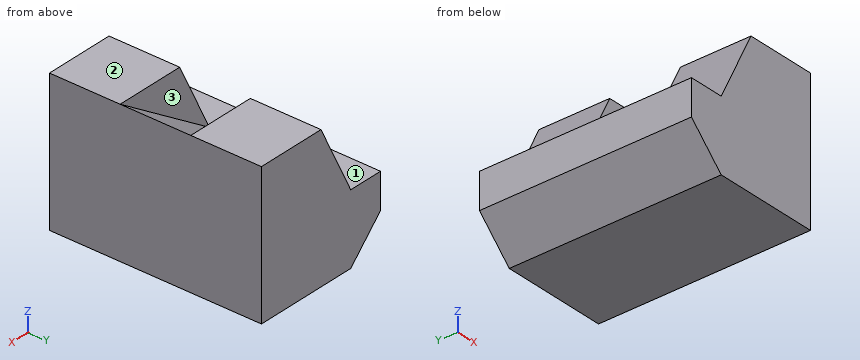
```python
from build123d import *

# Parameters (mm, degrees)
F1_DEPTH = 15
F2_DEPTH = 5


with BuildPart() as f1:
    # F0 (on Front) → F1 (new body, symmetric)
    with BuildSketch(Plane.XZ):
        Polygon((-15, 0), (0, 0), (0, 20), (-15, 10), (-20, 10), (-20, 5), align=None)
        Polygon((-15, 10), (0, 20), (-10, 20), align=None)
    extrude(amount=F1_DEPTH, both=True)

    # F0 (on Front) → F2 (cut, symmetric)
    with BuildSketch(Plane.XZ):
        Polygon((-15, 10), (0, 20), (-10, 20), align=None)
    extrude(amount=F2_DEPTH, both=True, mode=Mode.SUBTRACT)


solid = f1.part
```
Work out the finished part from the listing and answer in its coordinate system (mm). Face numbers are marked on the shaded views. A direction names the side the tool comes from. Round coordinates to 2 decimals unless told otherwise and drop trailing zeros. Write each loop counter-clockwise with the first axis right and the second up, starting at its lowest first coordinate (ties: lowest second). Pieces come first, ordered by that corner, then holes. Notation, with made-up numbers: (35.25, 56.25) - (88.25, 56.25) arc R9 cw to (88.25, 69.25) - close; hole circle Ø4 at (85, -27.75). An arc over 180 degrees is marked (long way). Return JSON: item names as keys, results as strings. Group by question number.
Q1. For the marked faces 1, 2 and 3, determine the directions among +Z, -Z, +X, -X, +Y, -Y from which every point of the face is accessible in a straight line to the end or side of a thin tool.
Q2. Find the intervals of material crossed by L1, parallel to Y at x = -11.5, z = 15.5; L2, parallel to Z at x = -16.75, y = -11; L3, parallel to X at y = -4.5, z = 15.5, in increasing order.
Q3. The part is cut by section D-D on y = -2.75. Write down the section's boundary in (x, z), then the cut area to 4 significant figures.
Q4. The part is cut by section C-C on x = -4.5. Write down the section's boundary in (y, z).
Q5. The part is cut by section B-B on z = 12. Write down the section's boundary in (x, y), then the cut area to 3 significant figures.
Q6. The part is cut by section A-A on y = -8.25. Write down the section's boundary in (x, z).
Q7. Each of these flat-tipped pins is pushed along its axis until it touches: pin 1 Ø4 at (y, z) = (0, 2.5) entering from -X; pin 2 Ø4 at (x, y) = (-18, -6) entering from +Z; pin 3 Ø5 at (x, y) = (-15, -0.5) entering from +Z; pin 4 Ø1.5 at (x, z) = (-14.5, 13.5) entering from +Y. Where does it stop, or does it pass through?
Solved:
{
 "1": {"face 1": "+Z, -X, +Y, -Y", "face 2": "+Z, +X, -X, +Y, -Y", "face 3": "+Z, -X"},
 "2": {"L1": "-15 to -5, 5 to 15", "L2": "1.75 to 10", "L3": "-6.75 to 0"},
 "3": {"outline": "(-20, 5) - (-15, 0) - (0, 0) - (0, 20) - (-15, 10) - (-20, 10) - close", "area": "262.5 mm²"},
 "4": {"outline": "(-15, 0) - (15, 0) - (15, 20) - (5, 20) - (5, 17) - (-5, 17) - (-5, 20) - (-15, 20) - close"},
 "5": {"outline": "(-14, -15) - (0, -15) - (0, 15) - (-14, 15) - (-14, 5) - (-12, 5) - (-12, -5) - (-14, -5) - close", "area": "400 mm²"},
 "6": {"outline": "(-20, 5) - (-15, 0) - (0, 0) - (0, 20) - (-10, 20) - (-15, 10) - (-20, 10) - close"},
 "7": {"pin 1": "x = -19.5", "pin 2": "z = 10", "pin 3": "z = 11.67", "pin 4": "through"}
}
